Answer from the drawing. Dimensions are ordinates in mm from the lowest x, y and z of the part. A direction names the side the tool comes from. Round coordinates to 2 decimals unless told otherwise and drop trailing zeros. Write each loop counter-clockwise with the first axis right and the second up, starting at its lowest first coordinate (ties: lowest second). Pieces come first, ordered by that corner, then holes. Notation, with made-up numbers: M 57.5,-21.75 L 68.5,-21.75 A17 cw 68.5,-11.75 Z; hole C 60.5,21 d8. An arc over 180 degrees is marked long. One line per item, written item: value. Start each with the question number.
(1) Section C-C (y = 799.5) is taken. Determine the outline of the cut face in (x, z), plus the area to 3 significant figures.
(2) For a pull along Y with two mould halves and no side action, classify the marked faces 1, 2, 3 and 4 as released by +Y, released by -Y, zero draft, split by the parting line, or undercut.
(3) Given P1, Ø2, axis at x = 257, z = 618.5, coming from the -Y side, flat-ended and moving along its own axis, determine where the tip first touches the part or whether it passes through.
(4) Consider probe 1 along Y at (x, z) = (335.5, 699.5); probe 2 along Z at (x, y) = (132.5, 58.5); probe 3 along Z at (x, y) = (419, 273.5). Determine where each line is inside the solid, lowest interval first.
(5) Section B-B (x = 83) is taken. Determine the outline of the cut face in (y, z).
(6) Section A-A (z = 579) is taken. Determine the outline of the cut face in (x, y), plus the area to 4 significant figures.
(7) Section D-D (y = 380.5) is taken. Determine the outline of the cut face in (x, z), plus the area to 4 significant figures.
(8) For the marked faces 5, 6 and 7, determine the directions among +Z, -Z, +X, -X, +Y, -Y from which every point of the face is accessible in a straight line to the end or side of a thin tool.
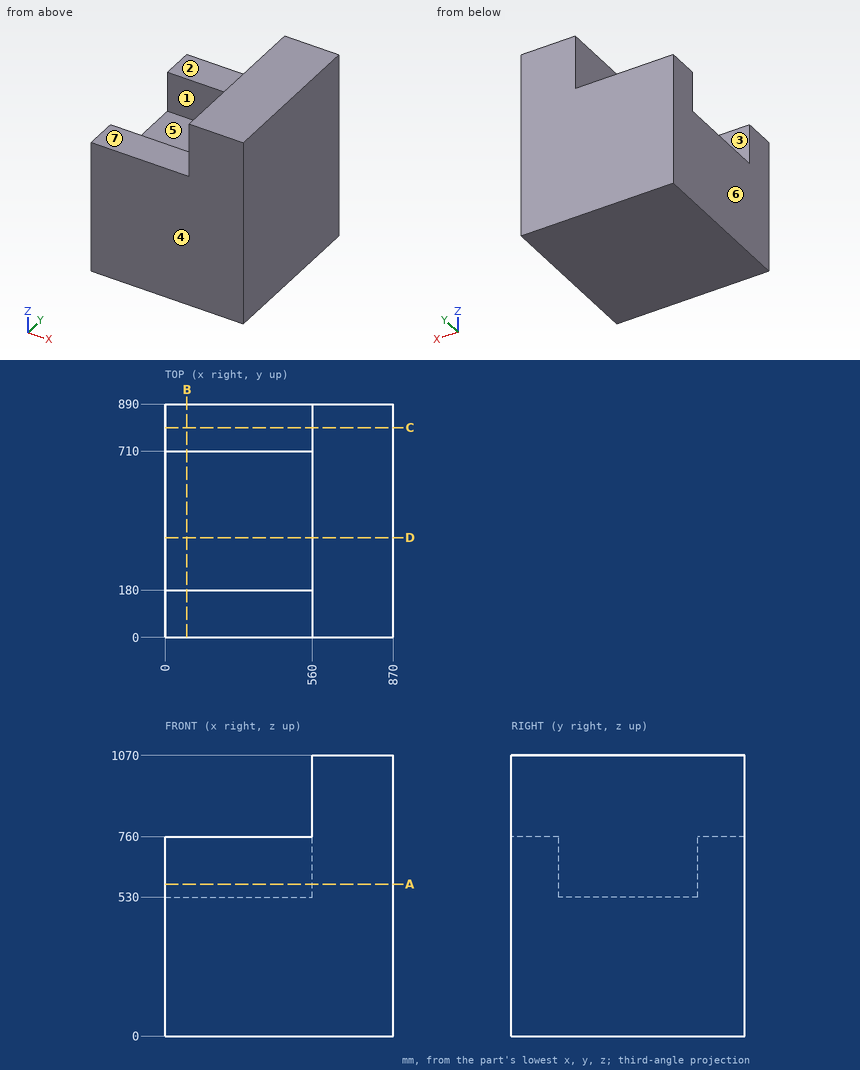
Recorded:
1. outline: M 0,0 L 870,0 L 870,1070 L 560,1070 L 560,760 L 0,760 Z
1. area: 757,000 mm2
2. face 1: undercut
2. face 2: zero draft
2. face 3: undercut
2. face 4: released by -Y
3. P1: stops at y = 0
4. probe 1: y = 0 to 180, 710 to 890
4. probe 2: z = 0 to 760
4. probe 3: z = 0 to 530
5. outline: M 0,0 L 890,0 L 890,760 L 710,760 L 710,530 L 180,530 L 180,760 L 0,760 Z
6. outline: M 0,0 L 870,0 L 870,890 L 0,890 L 0,710 L 560,710 L 560,180 L 0,180 Z
6. area: 477,500 mm2
7. outline: M 0,0 L 870,0 L 870,1070 L 560,1070 L 560,530 L 0,530 Z
7. area: 628,500 mm2
8. face 5: +Z, -X
8. face 6: +Z, -Z, -X, +Y, -Y
8. face 7: +Z, -X, +Y, -Y
